from build123d import *

# Parameters (mm, degrees)
F0_W     = 120
F0_H     = 380
F1_DEPTH = 60
F2_W     = 50
F2_H     = 340
F3_DEPTH = 30
F4_T     = -2.5
F5_W     = 120
F5_H     = 3
F6_DEPTH = 25
F8_DEPTH = 25


with BuildPart() as f1:
    # F0 (on Front) → F1 (new body)
    with BuildSketch(Plane.XZ):
        with Locations((60, 190)):
            Rectangle(F0_W, F0_H)
    extrude(amount=F1_DEPTH)

    # F2 (on face) → F3 (cut)
    with BuildSketch(Plane.XZ.offset(60)):
        with Locations((145, 190)):
            Rectangle(F2_W, F2_H)
        with Locations((95, 190)):
            Rectangle(F2_W, F2_H)
    extrude(amount=-F3_DEPTH, mode=Mode.SUBTRACT)

    # F4
    f4_openings = [f1.faces().sort_by_distance(p)[0] for p in [
        (95, -45, 20),
        (95, -30, 190),
        (70, -45, 190),
        (95, -45, 360),
    ]]
    offset(amount=F4_T, openings=f4_openings)

    # F5 (on face) → F6 (join)
    with BuildSketch(Plane.XY.offset(380)):
        with Locations((60, -1.5)):
            Rectangle(F5_W, F5_H)
    extrude(amount=F6_DEPTH)

    # F7 (on face) → F8 (cut)
    with BuildSketch(Plane.XZ.offset(3)):
        with BuildLine():
            ThreePointArc((64.880804, 395.873971), (63.476993, 399.347791), (60.053833, 400.870976))
            ThreePointArc((60.053833, 400.870976), (56.406984, 399.47016), (54.880804, 395.873971))
            Line((54.880804, 395.873971), (44.880804, 395.873971))
            ThreePointArc((44.880804, 395.873971), (41.130804, 392.123971), (44.880804, 388.373971))
            Line((44.880804, 388.373971), (74.880804, 388.373971))
            ThreePointArc((74.880804, 388.373971), (78.630804, 392.123971), (74.880804, 395.873971))
            Line((74.880804, 395.873971), (64.880804, 395.873971))
        make_face()
    extrude(amount=-F8_DEPTH, mode=Mode.SUBTRACT)


solid = f1.part
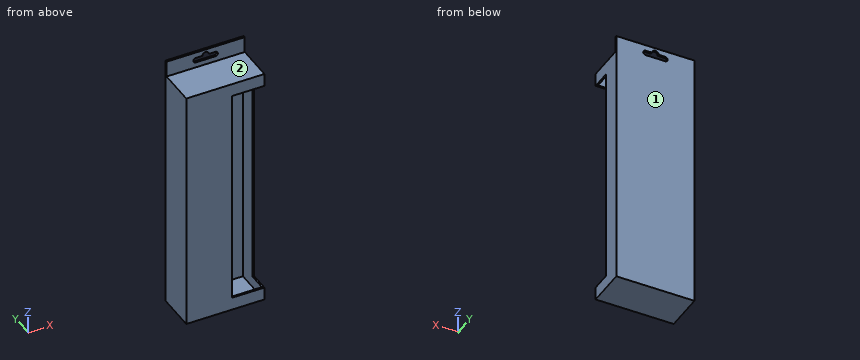
The listing builds one solid part. Answer for the finished solid, in the listing's coordinates (mm). Face numbers are marked on the shaded views. A direction names the side the tool comes from. Round coordinates to 2 decimals unless told otherwise and drop trailing zeros. Loops run counter-clockwise (first coordinate to the right, second up) from the corner with the lowest first, then second, coordinate; pieces in that order, holes last. Notation, with made-up numbers: M -21,89.25 L -14,89.25 A28 ccw -14,124.25 Z; hole C 8,-21 d8. An arc over 180 degrees is marked long. Write each question's results on one line, items separated by ' | '. Start each with the question number.
1) Straight lines are drawn through the part: probe 1 along Z at (x, y) = (35.5, -43.5); probe 2 along X at (y, z) = (-42.5, 368); probe 3 along Y at (x, z) = (52, 256). For each, find the intervals that lie inside material, in ascending order.
2) Find section C-C on z = 218. Write down the section's boundary in (x, y).
3) Find section B-B on x = 14. Write down the section's boundary in (y, z).
4) Find section A-A on y = -14.5. Write down the section's boundary in (x, z), plus the area to 4 significant figures.
5) Each of these flat-tipped pins is pushed along its axis until it touches: pin 1 (0.8 mm diameter, centred on y = -58.5, z = 213, fed in from +X); pin 2 (6 mm diameter, centred on x = 72.5, y = -8.5, fed in from +Z); pin 3 (20 mm diameter, centred on x = 58.5, z = 391.5, fed in from -Y). Where does it stop, or does it pass through?
6) Find section D-D on y = -34.5. Write down the section's boundary in (x, z).
7) Which of the six approach directions +Z, -Z, +X, -X, +Y, -Y give full straight-line access (tool end or side, diameter ignored) to the marked faces 1 and 2?
Final values:
1) probe 1: 0 to 2.5, 377.5 to 380 | probe 2: 0 to 2.5, 117.5 to 120 | probe 3: -60 to -57.5, -2.5 to 0
2) outline: M 0,-60 L 70,-60 L 70,-57.5 L 2.5,-57.5 L 2.5,-2.5 L 117.5,-2.5 L 117.5,-30 L 120,-30 L 120,0 L 0,0 Z
3) outline: M -60,0 L 0,0 L 0,405 L -3,405 L -3,380 L -60,380 Z; hole M -57.5,2.5 L -2.5,2.5 L -2.5,377.5 L -57.5,377.5 Z
4) outline: M 0,0 L 120,0 L 120,380 L 0,380 Z; hole M 2.5,2.5 L 117.5,2.5 L 117.5,377.5 L 2.5,377.5 Z | area: 2,475 mm²
5) pin 1: x = 70 | pin 2: z = 380 | pin 3: y = -3
6) outline: M 0,0 L 120,0 L 120,20 L 117.5,20 L 117.5,2.5 L 2.5,2.5 L 2.5,377.5 L 117.5,377.5 L 117.5,360 L 120,360 L 120,380 L 0,380 Z
7) face 1: +Z, -Z, +X, -X, +Y | face 2: +Z, +X, -X, -Y
